The listing builds one solid part. Answer for the finished solid, in the listing's coordinates (mm). A direction names the side the tool comes from. Coordinates: 2 decimals unless noted, no trailing zeros. Order: outer loops, then holes, each group sorted by start corner. A loop starts at its lowest first (then second) coordinate and runs counter-clockwise, first axis right, second up. Notation, with made-up numbers: (-27, 73.5) -> (12, 73.5) arc R11 cw to (12, 90.5) -> close; hole circle Ø10 at (71.25, -22). An arc over 180 degrees is marked (long way). Write each question's results on one line, items separated by ' | '. Start each with the question number.
(1) Straight lines are drawn through the part: L1, parallel to Y at x = 55.25, z = 50.65; L2, parallel to Y at x = 40.75, z = 47.5; L3, parallel to Y at x = 43.5, z = 37.5. For each, find the intervals that lie inside material, in ascending order.
(2) Given pin 1 (6 mm diameter, centred on x = 51.5, y = 9, fed in from -Z); pin 2 (3 mm diameter, centred on x = 43, z = 51, fed in from +Y); pin 3 (1 mm diameter, centred on x = 64, y = 5.5, fed in from +Z); pin 4 (5.5 mm diameter, centred on x = 45, z = 43, fed in from +Y), each flat-ended and moving along its own axis, determine where each tip first touches the part or whether it passes through.
(3) A tool of negligible diameter and unlimited length cuts with its end or side. For faces 1 (the face through (28.3, 7, 50)), 2 (the face through (34, 14, 47)), 3 (the face through (29.4, 6, 50)), 4 (the face through (67, 6, 42)), 5 (the face through (68, 8, 50)), from which of +Z, -Z, +X, -X, +Y, -Y can it reach the whole face along a straight path? Write none if from no direction.
(4) The part is cut by section A-A, the plane z = 40. Give the vertices of the cut face in (x, y), then the cut area to 3 significant figures.
(5) The part is cut by section D-D, the plane y = 6. Give the vertices of the cut face in (x, z).
(6) Determine the mould class of faces 6 (the face through (38.552, 10.597, 50.265)), 7 (the face through (35, 10, 47)), 8 (the face through (42, 10, 52.8)) for opening direction Y: +Y half, -Y half, draft (parallel to the pull), parting line (faces both ways), or undercut.
(7) The part is cut by section C-C, the plane z = 49.25. Give the vertices of the cut face in (x, y).
(8) The part is cut by section B-B, the plane x = 34. Give the vertices of the cut face in (y, z).
```python
from build123d import *

# Parameters (mm, degrees)
PAD063_DEPTH    = 42
SKETCH118_R     = 1
POCKET024_DEPTH = 2
POCKET025_DEPTH = 2
SKETCH120_R     = 2.2
SKETCH120_R_2   = 1
PAD070_DEPTH    = 5


with BuildPart() as part:
    # Sketch102 → Pad063 (new body)
    with BuildSketch(Plane.YZ):
        Polygon((5, -11), (7, -11), (7, -2), (16, -2), (16, 0), (5, 0), align=None)
    extrude(amount=PAD063_DEPTH)

    # Sketch118 → Pocket024 (cut)
    with BuildSketch(Plane(origin=(0, 5, 0), x_dir=(1, 0, 0), z_dir=(0, 0, 1))):
        with Locations((13.75, 5.5)):
            Circle(SKETCH118_R)
        with Locations((28.25, 5.5)):
            Circle(SKETCH118_R)
        Polygon((2, 9), (2, 2), (9, 2), align=None)
        Polygon((4, 9), (11, 9), (11, 2), align=None)
        Polygon((31, 9), (31, 2), (38, 2), align=None)
        Polygon((33, 9), (40, 9), (40, 2), align=None)
        Polygon((16.5, 9), (16.5, 2), (23.5, 2), align=None)
        Polygon((18.5, 9), (25.5, 9), (25.5, 2), align=None)
    extrude(amount=-POCKET024_DEPTH, mode=Mode.SUBTRACT)

    # Sketch119 → Pocket025 (cut)
    with BuildSketch(Plane.XZ.offset(-5)):
        Polygon((2, -3), (10, -3), (2, -9), align=None)
        Polygon((12, -3), (4, -9), (12, -9), align=None)
        Polygon((30, -3), (38, -3), (30, -9), align=None)
        Polygon((40, -3), (32, -9), (40, -9), align=None)
        Polygon((16, -3), (24, -3), (16, -9), align=None)
        Polygon((26, -3), (18, -9), (26, -9), align=None)
    extrude(amount=-POCKET025_DEPTH, mode=Mode.SUBTRACT)

    # Sketch120 → Pad070 (join)
    with BuildSketch(Plane.XY):
        with Locations((13.75, 10.5)):
            Circle(SKETCH120_R)
        with Locations((13.75, 10.5)):
            Circle(SKETCH120_R_2, mode=Mode.SUBTRACT)
        with Locations((28.25, 10.5)):
            Circle(SKETCH120_R)
        with Locations((28.25, 10.5)):
            Circle(SKETCH120_R_2, mode=Mode.SUBTRACT)
        Polygon((0, 8), (1.3, 8), (1.3, 6.4), (2.4, 6.4), (2.4, 5), (0, 5), align=None)
        Polygon((42, 5), (42, 8), (40.7, 8), (40.7, 6.4), (39.6, 6.4), (39.6, 5), align=None)
    extrude(amount=PAD070_DEPTH)


with BuildPart() as part_1:
    # Body095 placement: moved
    add(part.part.moved(Location((27, 0, 47.8))))


solid = part_1.part
```
Established:
1) L1: y = 8.3 to 9.5, 11.5 to 12.7 | L2: y = 5 to 9.5, 11.5 to 16 | L3: y = 5 to 7
2) pin 1: stops at z = 36.8 | pin 2: stops at y = 12.57 | pin 3: stops at z = 47.8 | pin 4: stops at y = 7
3) face 1: +Z, +Y | face 2: +Z, -Z | face 3: +Z, +Y, -Y | face 4: +Y, -Y | face 5: +Z, +X, -X, +Y
4) outline: (27, 5) -> (29, 5) -> (29, 7) -> (27, 7) -> close; (30.6, 5) -> (32.6, 5) -> (32.6, 7) -> (30.6, 7) -> close; (39, 5) -> (43, 5) -> (43, 7) -> (39, 7) -> close; (44.6, 5) -> (46.6, 5) -> (46.6, 7) -> (44.6, 7) -> close; (53, 5) -> (57, 5) -> (57, 7) -> (53, 7) -> close; (58.6, 5) -> (60.6, 5) -> (60.6, 7) -> (58.6, 7) -> close; (67, 5) -> (69, 5) -> (69, 7) -> (67, 7) -> close | area: 36.0 mm^2
5) outline: (27, 36.8) -> (69, 36.8) -> (69, 52.8) -> (66.6, 52.8) -> (66.6, 47.8) -> (29.4, 47.8) -> (29.4, 52.8) -> (27, 52.8) -> close; hole (29, 38.8) -> (37, 44.8) -> (29, 44.8) -> close; hole (31, 38.8) -> (39, 38.8) -> (39, 44.8) -> close; hole (43, 38.8) -> (51, 44.8) -> (43, 44.8) -> close; hole (45, 38.8) -> (53, 38.8) -> (53, 44.8) -> close; hole (57, 38.8) -> (65, 44.8) -> (57, 44.8) -> close; hole (59, 38.8) -> (67, 38.8) -> (67, 44.8) -> close
6) face 6: parting line | face 7: undercut | face 8: draft
7) outline: (27, 5) -> (29.4, 5) -> (29.4, 6.4) -> (28.3, 6.4) -> (28.3, 8) -> (27, 8) -> close; circle Ø4.4 at (40.75, 10.5); circle Ø4.4 at (55.25, 10.5); (66.6, 5) -> (69, 5) -> (69, 8) -> (67.7, 8) -> (67.7, 6.4) -> (66.6, 6.4) -> close; hole circle Ø2 at (40.75, 10.5); hole circle Ø2 at (55.25, 10.5)
8) outline: (5, 36.8) -> (7, 36.8) -> (7, 38.8) -> (5, 38.8) -> close; (5, 41.05) -> (7, 41.05) -> (7, 42.55) -> (5, 42.55) -> close; (5, 44.8) -> (7, 44.8) -> (7, 47.8) -> (5, 47.8) -> close; (9, 45.8) -> (11, 45.8) -> (11, 47.8) -> (9, 47.8) -> close; (14, 45.8) -> (16, 45.8) -> (16, 47.8) -> (14, 47.8) -> close
